The model under review builds one solid part; all positions refer to its coordinate system, in mm. A direction names the side the tool comes from. Give positions to 0.01 mm unless a question says otherwise; leave off trailing zeros. Loops run counter-clockwise (first coordinate to the right, second up) from the corner with the lowest first, then second, coordinate; pieces in that order, holes last. Notation, with made-up numbers: M 6.25,56 L 14.25,56 A25 ccw 14.25,81 Z; hole C 22.5,53.25 d2. An arc over 180 degrees is marked long. Write item = value, one per line. Start each with the question number.
1. We need section D-D on y = 28. Give the boundary of the cut face in (x, z), then the cut area to 3 significant figures.
2. Wall thickness on line 1 along Y through (x, z) = (-21.5, -3.5); line 2 along Y through (x, z) = (-8, 9); line 3 along Z through (x, y) = (11.5, 58.5): over which ranges is each line inside the solid? List them lowest first. Write a range as from..to.
3. We need section B-B on x = 0. Give the boundary of the cut face in (y, z).
4. We need section A-A on z = 6. Give the boundary of the cut face in (x, y), then the cut area to 3 significant figures.
5. Draft analysis for pull direction X (two halves, no side actions). For faces 5 (the face through (-11.467, 4.056, 19.686)), 6 (the face through (3, -4, -3)), 7 (the face through (14.985, 93.323, 0.66)), state which applies: pulls with the +X half, pulls with the -X half, needs draft (parallel to the pull), parting line crosses it, or undercut.
6. For pin 1 (4 mm diameter, centred on x = -3, y = 77.5, fed in from -Z); pin 2 (3 mm diameter, centred on x = 5.5, y = 39, fed in from -Z); pin 3 (4 mm diameter, centred on y = 5, z = -5, fed in from -X), all flat-tipped, find the tip position at first contact; note any pin that passes through.
7. For faces 1 (the face through (13, 5, 32)), 2 (the face through (7, 87.9, -15)), 3 (the face through (-0.867, -1.972, -3.905)), 4 (the face through (-7.493, -10.902, 0.33)), list the 3-axis set-ups (+Z, -Z, +X, -X, +Y, -Y) from which the entire face can be reached by the end or side of a thin tool; tool diameter is ignored.
8. We need section C-C on z = -11. Give the boundary of the cut face in (x, y).
from build123d import *

# Parameters (mm, degrees)
F0_R      = 33.75
F1_DEPTH  = 87.9
F2_R      = 15
F3_DEPTH  = 11
F4_R      = 4
F5_DEPTH  = 24
F6_D      = 4
F6_DEPTH  = 8
F6_TIP    = 1.2017212381
F8_R      = 7.5
F9_DEPTH  = 14
F12_DEPTH = 13.5


with BuildPart() as f1:
    # F0 (on Front) → F1 (new body)
    with BuildSketch(Plane.XZ):
        Circle(F0_R)
    extrude(amount=-F1_DEPTH)

    # F2 (on face) → F3 (join)
    with BuildSketch(Plane(origin=(0, 87.9, 0), x_dir=(-1, 0, 0), z_dir=(0, 1, 0))):
        Circle(F2_R)
    extrude(amount=F3_DEPTH)

    # F4 (on face) → F5 (join)
    with BuildSketch(Plane.XZ):
        Circle(F4_R)
    extrude(amount=F5_DEPTH)

    # F6
    with Locations(Plane.XZ):
        with Locations((20.7846096908, 0), (-10.3923048454, 18), (-10.3923048454, -18)):
            Hole(F6_D / 2, depth=F6_DEPTH)
            with Locations((0, 0, -(F6_DEPTH + F6_TIP / 2))):  # 118° drill point
                Cone(0, F6_D / 2, F6_TIP, mode=Mode.SUBTRACT)

    # F8 (on offset) → F9 (join)
    with BuildSketch(Plane.XZ.offset(4)):
        Circle(F8_R)
    extrude(amount=F9_DEPTH)

    # F11 (on offset) → F12 (join)
    with BuildSketch(Plane.XZ.offset(-5)):
        with BuildLine():
            Line((20.2615004909, 26.9913708036), (21.6578633283, 30.5492955083))
            Line((21.6578633283, 30.5492955083), (4.9021042855, 37.1253535145))
            Line((4.9021042855, 37.1253535145), (3.5057414481, 33.5674288098))
            ThreePointArc((3.5057414481, 33.5674288098), (12.3301087616, 31.4170482052), (20.2615004909, 26.9913708036))
        make_face()
    extrude(amount=-F12_DEPTH)


solid = f1.part
Final values:
q1.outline = C 0,0 d67.5
q1.area = 3,580 mm²
q2.line_1 = 0..87.9
q2.line_2 = 0..98.9
q2.line_3 = -31.73..31.73
q3.outline = M -24,-4 L -18,-4 L -18,-7.5 L -4,-7.5 L -4,-4 L 0,-4 L 0,-33.75 L 87.9,-33.75 L 87.9,-15 L 98.9,-15 L 98.9,15 L 87.9,15 L 87.9,33.75 L 0,33.75 L 0,4 L -4,4 L -4,7.5 L -18,7.5 L -18,4 L -24,4 Z
q4.outline = M -33.21,0 L 33.21,0 L 33.21,87.9 L 13.75,87.9 L 13.75,98.9 L -13.75,98.9 L -13.75,87.9 L -33.21,87.9 Z; M -4.5,-18 L 4.5,-18 L 4.5,-4 L -4.5,-4 Z
q4.area = 6,270 mm²
q5.face_5 = undercut
q5.face_6 = needs draft
q5.face_7 = parting line crosses it
q6.pin_1 = -33.74
q6.pin_2 = -33.51
q6.pin_3 = -33.62
q7.face_1 = +Z, +X, -Y
q7.face_2 = +Y
q7.face_3 = none
q7.face_4 = -Y
q8.outline = M -31.91,0 L 31.91,0 L 31.91,87.9 L 10.2,87.9 L 10.2,98.9 L -10.2,98.9 L -10.2,87.9 L -31.91,87.9 Z
